Autodesk Inventor part; units mm, degrees
ref_plane "YZ Plane" through (0, 0, 0) normal (1, 0, 0) x (0, 1, 0)
ref_plane "XZ Plane" through (0, 0, 0) normal (0, 1, 0) x (-1, 0, 0)
ref_plane "XY Plane" through (0, 0, 0) normal (0, 0, 1) x (1, 0, 0)
sketch "Boceto1" plane through (0, 0, 0) normal (0, 1, 0) x (-1, 0, 0)
  line L0 (1.5588, -2.7) -> (-1.5588, -2.7)
  line L1 (-1.5588, -2.7) -> (-3.1177, 0)
  line L2 (-3.1177, 0) -> (-1.5588, 2.7)
  line L3 (-1.5588, 2.7) -> (1.5588, 2.7)
  line L4 (1.5588, 2.7) -> (3.1177, 0)
  line L5 (3.1177, 0) -> (1.5588, -2.7)
  line L6 (3.4064, 0) -> (1.7032, 2.95)
  line L7 (1.7032, 2.95) -> (-1.7032, 2.95)
  line L8 (-1.7032, 2.95) -> (-3.4064, 0)
  line L9 (-3.4064, 0) -> (-1.7032, -2.95)
  line L10 (-1.7032, -2.95) -> (1.7032, -2.95)
  line L11 (1.7032, -2.95) -> (3.4064, 0)
  circle A0 centre (0, 0) radius 7.5
  dimension "d0" = 5.4
  dimension "d1" = 0.25
  dimension "d2" = 15
extrude "Extrusión1" add sketch "Boceto1" along normal blind 6 contours L0 L1 L2 L3 L4 L5 | L11 L10 L9 L8 L7 L6 | A0
sketch "Boceto2" plane through (0, 6, 0) normal (0, 1, 0) x (1, 0, 0)
  line L0 (-3.1177, 0) -> (-1.5588, 2.7)
  line L1 (-1.5588, 2.7) -> (1.5588, 2.7)
  line L2 (1.5588, 2.7) -> (3.1177, 0)
  line L3 (3.1177, 0) -> (1.5588, -2.7)
  line L4 (1.5588, -2.7) -> (-1.5588, -2.7)
  line L5 (-1.5588, -2.7) -> (-3.1177, 0)
  line L6 (-3.4064, 0) -> (-1.7032, 2.95)
  line L7 (-1.7032, 2.95) -> (1.7032, 2.95)
  line L8 (1.7032, 2.95) -> (3.4064, 0)
  line L9 (3.4064, 0) -> (1.7032, -2.95)
  line L10 (1.7032, -2.95) -> (-1.7032, -2.95)
  line L11 (-1.7032, -2.95) -> (-3.4064, 0)
  point P0 (0, 0)
  point P1 (0, 0)
  dimension "d5" = 5.4
  dimension "d6" = 0.25
extrude "Extrusión2" cut sketch "Boceto2" against normal blind 4 contours L0 L1 L2 L3 L4 L5 | L6 L7 L8 L9 L10 L11
sketch "Boceto3" plane through (0, 2, 0) normal (0, 1, 0) x (1, 0, 0)
  circle A0 centre (0, 0) radius 7.5
hole "Agujero1" at (0, 2, 0) direction (0, -1, 0) diameter 3 end through all
properties part number "Cabeza_Tornillos"
Here's how the part is built. I have some questions about the finished solid (model axes, mm). A direction names the side the tool comes from. Round coordinates to 2 decimals unless told otherwise and drop trailing zeros. Loops run counter-clockwise (first coordinate to the right, second up) from the corner with the lowest first, then second, coordinate; pieces in that order, holes last. Notation, with made-up numbers: (71, -31) -> (113, -31) arc R20 cw to (113, 8) -> close; hole circle Ø2 at (7, -34.5). An arc over 180 degrees is marked (long way). Write each question's results on one line, items separated by ' | '.
(1) We'd pull the mould along X, two halves only. Please class faces 1 (the face through (7.493, 2.958, -0.33)), 2 (the face through (-0.07, 0.99, -1.5)), 3 (the face through (0, 0, -2)): released by +X, released by -X, zero draft, split by the parting line, or undercut.
Worked answers:
face 1: split by the parting line | face 2: undercut | face 3: zero draft
(2) If we section it at D-D, the plane y = 1: List the corners of the cut face in (x, z) for me, then the cut area to 3 significant figures.
Worked answers:
outline: circle Ø15 at (0, 0); hole circle Ø3 at (0, 0) | area: 170 mm2
(3) If we section it at C-C, the plane z = -0.25: List the corners of the cut face in (x, y) for me, then the cut area to 3 significant figures.
Worked answers:
outline: (-7.5, 0) -> (-1.48, 0) -> (-1.48, 2) -> (-3.26, 2) -> (-3.26, 6) -> (-7.5, 6) -> close; (1.48, 0) -> (7.5, 0) -> (7.5, 6) -> (3.26, 6) -> (3.26, 2) -> (1.48, 2) -> close | area: 57.9 mm2
(4) If I drill on L1, parallel to Z at x = 0, y = 0.85; L2, parallel to Z at x = 2, y = 3.9; L3, parallel to Y at x = -2.5, z = 0.25, over which ranges is the centre line in solid material (lowest first)?
Worked answers:
L1: -7.5 to -1.5, 1.5 to 7.5 | L2: -7.23 to -2.44, 2.44 to 7.23 | L3: 0 to 2
(5) For faces 4 (the face through (0.1, 6, -3.2)), 5 (the face through (2.57, 4.03, 1.45)), which set-ups out of +Z, -Z, +X, -X, +Y, -Y let a thin tool reach every point of the face, with its end or its side?
Worked answers:
face 4: +Z, -Z, +X, -X, +Y | face 5: +Y
(6) For P1, Ø1.8, axis at x = -1, z = -1, coming from the +Y side; P2, Ø1, axis at y = 2, z = 4.5, coming from the -X side; P3, Ø3, axis at y = 4.5, z = -3, coming from the +X side, each with a flat end and sliding along its axis, tell me the tip position at first contact or that it passes through.
Worked answers:
P1: y = 2 | P2: x = -6.34 | P3: x = 7.35
(7) If we section it at B-B, the plane y = 4.25: List the corners of the cut face in (x, z) for me, then the cut area to 3 significant figures.
Worked answers:
outline: circle Ø15 at (0, 0); hole (-3.41, 0) -> (-1.7, -2.95) -> (1.7, -2.95) -> (3.41, 0) -> (1.7, 2.95) -> (-1.7, 2.95) -> close | area: 147 mm2
(8) If we section it at A-A, the plane x = 0: List the corners of the cut face in (y, z) for me.
Worked answers:
outline: (0, -7.5) -> (6, -7.5) -> (6, -2.95) -> (2, -2.95) -> (2, -1.5) -> (0, -1.5) -> close; (0, 1.5) -> (2, 1.5) -> (2, 2.95) -> (6, 2.95) -> (6, 7.5) -> (0, 7.5) -> close
